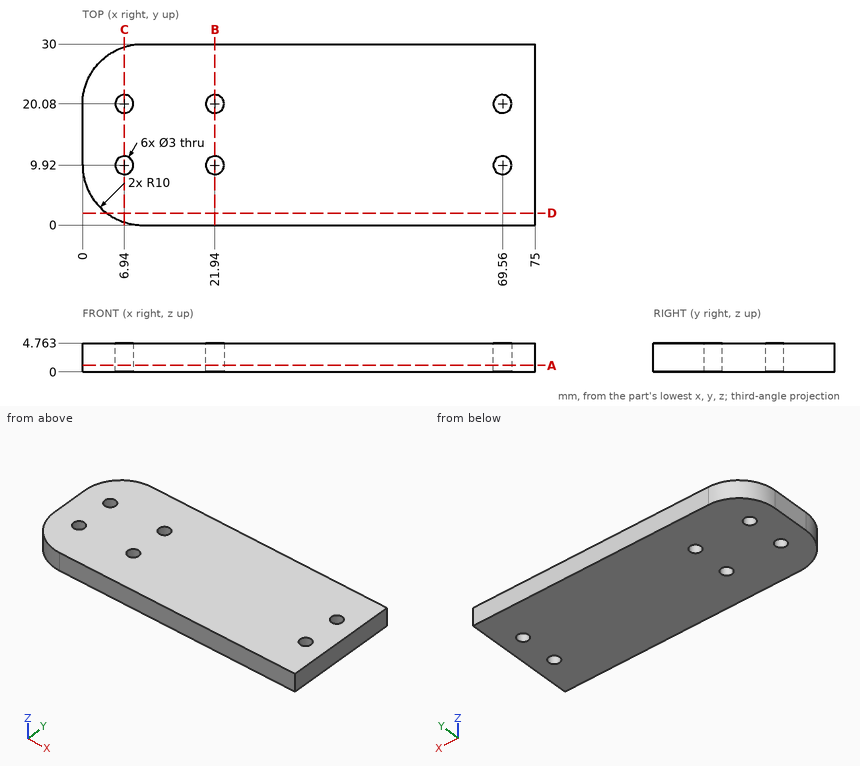
Could you check a few things on this drawing? It's one solid part, dimensions in mm from its lowest x, y, z. Give positions to 0.01 mm unless a question says otherwise; leave off trailing zeros. Order: outer loops, then holes, each group sorted by start corner. A loop starts at its lowest first (then second) coordinate and runs counter-clockwise, first axis right, second up. Notation, with made-up numbers: (-33.5, 27.5) - (-28.5, 27.5) arc R15 ccw to (-28.5, 49.5) - close; hole circle Ø7 at (34, 83). An arc over 180 degrees is marked (long way). One line per question, with ' | ' between items. Start each with the question number.
Item 1: I want a section at A-A on z = 1.1. Write out the boundary of the cut face in (x, y), then the cut area to 3 significant figures.
Item 2: I need wall thicknesses on probe 1 along Y at (x, z) = (69.56, 3.2); probe 2 along X at (y, z) = (10, 2.55); probe 3 along Y at (x, z) = (6.94, 3.45). Which ranges of each line are inside material? Lowest first, please. Write a range as [from, to].
Item 3: I want a section at C-C on x = 6.94. Write out the boundary of the cut face in (y, z), then the cut area to 3 significant figures.
Item 4: I want a section at B-B on x = 21.94. Write out the boundary of the cut face in (y, z).
Item 5: I want a section at D-D on y = 2. Write out the boundary of the cut face in (x, z), then the cut area to 3 significant figures.
Item 6: I'm going to push flat-ended pins straight in: pin 1 Ø3.5 at (x, y) = (6.94, 20.08) entering from -Z; pin 2 Ø2 at (y, z) = (4, 4) entering from -X. Where does each tip first touch, or does it pass through?
Verdict:
1) outline: (0, 10) arc R10 ccw to (10, 0) - (75, 0) - (75, 30) - (10, 30) arc R10 ccw to (0, 20) - close; hole circle Ø3 at (6.94, 9.92); hole circle Ø3 at (6.94, 20.08); hole circle Ø3 at (21.94, 9.92); hole circle Ø3 at (21.94, 20.08); hole circle Ø3 at (69.56, 9.92); hole circle Ø3 at (69.56, 20.08) | area: 2,160 mm^2
2) probe 1: [0, 8.42], [11.42, 18.58], [21.58, 30] | probe 2: [0, 5.44], [8.44, 20.44], [23.44, 68.06], [71.06, 75] | probe 3: [0.48, 8.42], [11.42, 18.58], [21.58, 29.52]
3) outline: (0.48, 0) - (8.42, 0) - (8.42, 4.76) - (0.48, 4.76) - close; (11.42, 0) - (18.58, 0) - (18.58, 4.76) - (11.42, 4.76) - close; (21.58, 0) - (29.52, 0) - (29.52, 4.76) - (21.58, 4.76) - close | area: 110 mm^2
4) outline: (0, 0) - (8.42, 0) - (8.42, 4.76) - (0, 4.76) - close; (11.42, 0) - (18.58, 0) - (18.58, 4.76) - (11.42, 4.76) - close; (21.58, 0) - (30, 0) - (30, 4.76) - (21.58, 4.76) - close
5) outline: (4, 0) - (75, 0) - (75, 4.76) - (4, 4.76) - close | area: 338 mm^2
6) pin 1: z = 0 | pin 2: x = 1.34
